from build123d import *

# Parameters (mm, degrees)
SKETCH_1_W          = 55
SKETCH_1_H          = 28
SKETCH_1_R          = 5.1
SKETCH_1_R_2        = 1.6
EXTRUDE_1_DEPTH     = 3
SKETCH_2_R          = 1.6
CUT_EXTRUDE_1_DEPTH = 32.004031996
FILLET_1_R          = 2


with BuildPart() as part:
    # 草图1 → 凸台-拉伸1 (new body)
    with BuildSketch(Plane(origin=(0, 0, 0), x_dir=(1, 0, 0), z_dir=(0, 1, 0))):
        Rectangle(SKETCH_1_W, SKETCH_1_H)
        with Locations(Location((0, 0, 0), (0, 0, 270))):
            Circle(SKETCH_1_R, mode=Mode.SUBTRACT)
        with Locations(Location((5.656854249, 5.656854249, 0), (0, 0, 270))):
            Circle(SKETCH_1_R_2, mode=Mode.SUBTRACT)
        with Locations(Location((-5.656854249, -5.656854249, 0), (0, 0, 270))):
            Circle(SKETCH_1_R_2, mode=Mode.SUBTRACT)
        with Locations(Location((6.717514421, -6.717514421, 0), (0, 0, 270))):
            Circle(SKETCH_1_R_2, mode=Mode.SUBTRACT)
        with Locations(Location((-6.717514421, 6.717514421, 0), (0, 0, 270))):
            Circle(SKETCH_1_R_2, mode=Mode.SUBTRACT)
    extrude(amount=EXTRUDE_1_DEPTH)

    # 草图2 → 切除-拉伸1 (cut, through all)
    with BuildSketch(Plane(origin=(0, 3, 0), x_dir=(1, 0, 0), z_dir=(0, 1, 0))):
        with Locations(Location((-24.5, 11, 0), (0, 0, 270))):
            Circle(SKETCH_2_R)
        with Locations(Location((-24.5, -11, 0), (0, 0, 270))):
            Circle(SKETCH_2_R)
        with Locations(Location((24.5, 11, 0), (0, 0, 90))):
            Circle(SKETCH_2_R)
        with Locations(Location((24.5, -11, 0), (0, 0, 90))):
            Circle(SKETCH_2_R)
        with Locations((422.703102168, 0)):
            Circle(SKETCH_2_R)
        with Locations(Location((18.5, 0, 0), (0, 0, 270))):
            Circle(SKETCH_2_R)
        with Locations(Location((-18.5, 0, 0), (0, 0, 90))):
            Circle(SKETCH_2_R)
    extrude(amount=-CUT_EXTRUDE_1_DEPTH, mode=Mode.SUBTRACT)

    # 圆角1
    fillet_1_edges = [part.edges().sort_by_distance(p)[0] for p in [
        (27.5, 1.5, 14),
        (-27.5, 1.5, 14),
        (-27.5, 1.5, -14),
        (27.5, 1.5, -14),
    ]]
    fillet(fillet_1_edges, radius=FILLET_1_R)


solid = part.part
Can you work these out from the model? Positions are in its coordinate system, mm. Round coordinates to 2 decimals unless told otherwise and drop trailing zeros. Order: outer loops, then holes, each group sorted by start corner. A loop starts at its lowest first (then second) coordinate and runs counter-clockwise, first axis right, second up. Notation, with made-up numbers: M 36,16.5 L 93,16.5 A23 cw 93,38.5 Z; hole C 30,48.25 d5. An arc over 180 degrees is marked long. Use a Markdown table: item, result.
1) I'm going to push a flat-ended pin straight in: P1, Ø8, axis at x = 0, z = 0, coming from the -Y side. Where does the tip first touch, or does it pass through?
Geometry says:
| item | result |
|---|---|
| P1 | passes through |
2) If we mould it in two halves opening along Z, with no side actions, what happens to faces 1 (the face through (-6, 0, 0)), 2 (the face through (7.01, 1.48, -4.8)), 3 (the face through (26.9, 1.52, 13.43)), 4 (the face through (23.42, 1.52, 12.18))? For each: +Z half, -Z half, draft (parallel to the pull), parting line (faces both ways), or undercut.
Geometry says:
| item | result |
|---|---|
| face 1 | draft |
| face 2 | undercut |
| face 3 | +Z half |
| face 4 | undercut |
3) If I drill on line 1 along X through (y, z) = (2, 11); line 2 along X through (y, z) = (1.25, 0); line 3 along Z through (x, y) = (-18.5, 1.6), over which ranges is the centre line in solid material (lowest first)?
Geometry says:
| item | result |
|---|---|
| line 1 | x = -27.5 to -26.1, -22.9 to 22.9, 26.1 to 27.5 |
| line 2 | x = -27.5 to -20.1, -16.9 to -5.1, 5.1 to 16.9, 20.1 to 27.5 |
| line 3 | z = -14 to -1.6, 1.6 to 14 |
4) Imagine slicing it at D-D (x = -24.5). List the corners of the cut face in (y, z) for me.
Geometry says:
| item | result |
|---|---|
| outline | M 0,-14 L 3,-14 L 3,-12.6 L 0,-12.6 Z; M 0,-9.4 L 3,-9.4 L 3,9.4 L 0,9.4 Z; M 0,12.6 L 3,12.6 L 3,14 L 0,14 Z |
5) Imagine slicing it at A-A (x = 0). List the corners of the cut face in (y, z) for me.
Geometry says:
| item | result |
|---|---|
| outline | M 0,-14 L 3,-14 L 3,-5.1 L 0,-5.1 Z; M 0,5.1 L 3,5.1 L 3,14 L 0,14 Z |
6) Imagine slicing it at C-C (z = -11). List the corners of the cut face in (x, y) for me, then the cut area to 3 significant figures.
Geometry says:
| item | result |
|---|---|
| outline | M -27.5,0 L -26.1,0 L -26.1,3 L -27.5,3 Z; M -22.9,0 L 22.9,0 L 22.9,3 L -22.9,3 Z; M 26.1,0 L 27.5,0 L 27.5,3 L 26.1,3 Z |
| area | 146 mm² |
7) Imagine slicing it at B-B (z = 0). List the corners of the cut face in (x, y) for me, then the cut area to 3 significant figures.
Geometry says:
| item | result |
|---|---|
| outline | M -27.5,0 L -20.1,0 L -20.1,3 L -27.5,3 Z; M -16.9,0 L -5.1,0 L -5.1,3 L -16.9,3 Z; M 5.1,0 L 16.9,0 L 16.9,3 L 5.1,3 Z; M 20.1,0 L 27.5,0 L 27.5,3 L 20.1,3 Z |
| area | 115 mm² |
